from build123d import *

# Parameters (mm, degrees)
F0_W     = 19.05
F0_H     = 50.8
F2_T     = -2.54
F4_ANGLE = 180


with BuildPart() as f1:
    # F0 (on Front) → F1 (revolve)
    with BuildSketch(Plane.XZ):
        with Locations((28.321, 29.9166932978)):
            Rectangle(F0_W, F0_H)
    revolve(axis=Axis((18.796, 0, 29.9166932978), (0, 0, -1)))

    # F2
    f2_openings = [f1.faces().sort_by_distance(p)[0] for p in [
        (18.796, 0, 55.316693),
    ]]
    offset(amount=F2_T, openings=f2_openings)

    # F3 (on Right) → F4 (revolve)
    with BuildSketch(Plane.YZ):
        Polygon((-4.9335755283, 13.4986876266), (-3.0797308855, 9.639682645), (1.0932139292, 8.683026499), (4.4429463577, 11.3491007788), (4.4470495593, 15.6302971737), (1.1024337395, 18.3027874778), (-3.0723371717, 17.3541319833), align=None)
    revolve(axis=Axis((0, -0.516686556, 27.0530247144), (0, 1, 0)), revolution_arc=F4_ANGLE)


solid = f1.part
Verification items for the finished model (mm, model axes). A direction names the side the tool comes from. Give positions to 0.01 mm unless a question says otherwise; leave off trailing zeros. Write each loop counter-clockwise with the first axis right and the second up, starting at its lowest first coordinate (ties: lowest second). Pieces come first, ordered by that corner, then holes.
(1) Cross-section at D-D (y = 11). Enter the section's corners in (x, z).
(2) Access from +Z, -Z, +X, -X, +Y, -Y to the whole of each face (thin tool, end or side, straight path). Record for faces 4 (the face through (-9.94, -3.19, 26.83)), 5 (the face through (5.694, 10.046, 31.525)).
(3) Cross-section at C-C (x = 21). Enter the section's corners in (y, z), plus the area to 3 significant figures.
(4) Material ranges on line 1 (X direction, y = 0, z = 29.5); line 2 (Y direction, x = 19.5, z = 33.5); line 3 (X direction, y = 0, z = 30), recorded low to high.
(5) Cross-section at B-B (z = 24). State how many separate pieces and enclosed holes the cut face has, plus the area to 3 significant figures.
(6) Mould release check, pull along X, two halves, no side actions. Record for faces 1 (the face through (19, 0, 4.517)), 2 (the face through (-17.575, -2.355, 26.667)), 3 (the face through (0, -4, 14)): +X half, -X half, draft (parallel to the pull), parting line (faces both ways), or undercut.
(7) Gauge pin test, flat ends, axial feed: pin 1 (10 mm diameter, centred on y = -3, z = 46.5, fed in from -X); pin 2 (4 mm diameter, centred on x = 21.5, y = 1.5, fed in from +Z); pin 3 (6 mm diameter, centred on x = 6.5, z = 19, fed in from -Y); pin 4 (5 mm diameter, centred on x = -5, y = 8, fed in from -Z). Record the tip position at first contact, or that the pin passes through.
Worked out:
1. outline: (3.24, 4.52) - (34.35, 4.52) - (34.35, 55.32) - (31.11, 55.32) - (31.11, 7.06) - (6.48, 7.06) - (6.48, 55.32) - (3.24, 55.32) - close
2. face 4: -Y
2. face 5: +Z
3. outline: (-18.92, 4.52) - (18.92, 4.52) - (18.92, 55.32) - (16.36, 55.32) - (16.36, 7.06) - (-16.36, 7.06) - (-16.36, 55.32) - (-18.92, 55.32) - close
3. area: 343 mm2
4. line 1: x = -17.95 to -8.66, -0.25 to 2.29, 35.31 to 37.85
4. line 2: y = -19.04 to -16.49, 16.49 to 19.04
4. line 3: x = -17.88 to -8.5, -0.25 to 2.29, 35.31 to 37.85
5. separate pieces: 2
5. enclosed holes: 1
5. area: 352 mm2
6. face 1: draft
6. face 2: -X half
6. face 3: undercut
7. pin 1: stops at x = -10.03
7. pin 2: stops at z = 7.06
7. pin 3: stops at y = -16.63
7. pin 4: passes through
